```python
from build123d import *

# Parameters (mm, degrees)
F1_DEPTH = 60
F2_DEPTH = 40
F0_W     = 60
F0_H     = 20
F3_DEPTH = 20


with BuildPart() as f1:
    # F0 (on Top) → F1 (new body)
    with BuildSketch(Plane.XY):
        with BuildLine():
            Line((60, 60), (0, 60))
            ThreePointArc((0, 60), (30, 30), (60, 60))
        make_face()
    extrude(amount=F1_DEPTH)

    # F0 (on Top) → F2 (join)
    with BuildSketch(Plane.XY):
        with BuildLine():
            Line((0, 60), (0, 20))
            Line((0, 20), (60, 20))
            Line((60, 20), (60, 60))
            ThreePointArc((60, 60), (30, 30), (0, 60))
        make_face()
    extrude(amount=F2_DEPTH)

    # F0 (on Top) → F3 (join)
    with BuildSketch(Plane.XY):
        with Locations((30, 10)):
            Rectangle(F0_W, F0_H)
    extrude(amount=F3_DEPTH)


solid = f1.part
```
Could you check a few things on this model? Use its own coordinates, in mm. A direction names the side the tool comes from. Give positions to 0.01 mm unless a question says otherwise; leave off trailing zeros. Write each loop counter-clockwise with the first axis right and the second up, starting at its lowest first coordinate (ties: lowest second). Pieces come first, ordered by that corner, then holes. Notation, with made-up numbers: (55, -17.5) - (63, -17.5) arc R26 ccw to (63, 2.5) - close; hole circle Ø2 at (70, 35.25). An arc over 180 degrees is marked (long way). One line per item, written item: value. Start each with the question number.
Item 1: Imagine slicing it at C-C, the plane z = 28. List the corners of the cut face in (x, y) for me.
Item 2: I'm going to push flat-ended pins straight in: pin 1 (6 mm diameter, centred on x = 45, y = 12.5, fed in from +Z); pin 2 (2 mm diameter, centred on x = 7.5, z = 48.5, fed in from -Y). Where does each tip first touch, or does it pass through?
Item 3: Imagine slicing it at A-A, the plane x = 30. List the corners of the cut face in (y, z) for me.
Item 4: Imagine slicing it at B-B, the plane y = 12. List the corners of the cut face in (x, z) for me, and give its area (3 significant figures).
Item 5: Imagine slicing it at D-D, the plane x = 51. List the corners of the cut face in (y, z) for me, and give its area (3 significant figures).
Item 6: Please list where these lines run through material, in increasing order: line 1 (Z direction, x = 2.5, y = 13); line 2 (Y direction, x = 18, z = 31); line 3 (Z direction, x = 46, y = 29). Write a range as from..to.
Item 7: Which directions (+Z, -Z, +X, -X, +Y, -Y) give clear straight access to the entire face, cutting with the end or side of a thin tool? Please do faces 1 (the face through (0, 36, 20)), 2 (the face through (30, 10, 20)), 3 (the face through (30, 27, 40)).
Geometry says:
1. outline: (0, 20) - (60, 20) - (60, 60) - (0, 60) - close
2. pin 1: z = 20
2. pin 2: y = 39.08
3. outline: (0, 0) - (60, 0) - (60, 60) - (30, 60) - (30, 40) - (20, 40) - (20, 20) - (0, 20) - close
4. outline: (0, 0) - (60, 0) - (60, 20) - (0, 20) - close
4. area: 1,200 mm^2
5. outline: (0, 0) - (60, 0) - (60, 60) - (38.58, 60) - (38.58, 40) - (20, 40) - (20, 20) - (0, 20) - close
5. area: 2,430 mm^2
6. line 1: 0..20
6. line 2: 20..60
6. line 3: 0..40
7. face 1: +Z, -Z, -X, +Y, -Y
7. face 2: +Z, +X, -X, -Y
7. face 3: +Z, -Y
